```python
from build123d import *

# Parameters (mm, degrees)
SKETCH1_W           = 42.1
SKETCH1_H           = 42.1
BOSS_EXTRUDE1_DEPTH = 32.4
SKETCH2_W           = 17
SKETCH2_H           = 8.5
BOSS_EXTRUDE2_DEPTH = 7.9
BOSS_EXTRUDE3_DEPTH = 7.15
BOSS_EXTRUDE4_DEPTH = 7.2
SKETCH6_R           = 1.5
CUT_EXTRUDE1_DEPTH  = 7.2
CUT_EXTRUDE2_DEPTH  = 7.2
SKETCH9_R           = 6.55
BOSS_EXTRUDE5_DEPTH = 14.6
SKETCH11_R          = 9
BOSS_EXTRUDE6_DEPTH = 6.1
SKETCH12_W          = 17
SKETCH12_H          = 2.5
CUT_EXTRUDE3_DEPTH  = 6
CUT_EXTRUDE4_DEPTH  = 40


with BuildPart() as part:
    # Sketch1 → Boss-Extrude1 (new body)
    with BuildSketch(Plane.XY):
        with Locations((-21.05, 21.05)):
            Rectangle(SKETCH1_W, SKETCH1_H)
    extrude(amount=BOSS_EXTRUDE1_DEPTH)

    # Sketch2 → Boss-Extrude2 (add)
    with BuildSketch(Plane(origin=(0, 42.1, 0), x_dir=(1, 0, 0), z_dir=(0, 1, 0))):
        with Locations((-21.05, -4.25)):
            Rectangle(SKETCH2_W, SKETCH2_H)
    extrude(amount=BOSS_EXTRUDE2_DEPTH)

    # Sketch3 → Boss-Extrude3 (add)
    with BuildSketch(Plane(origin=(0, 0, 0), x_dir=(0, 0, -1), z_dir=(1, 0, 0))):
        Polygon((-32.4, 21.05), (-32.4, 29.05), (-30.8, 29.05), (-30.8, 21.05), (-30.8, 13.05), (-32.4, 13.05), align=None)
    extrude(amount=BOSS_EXTRUDE3_DEPTH)

    # Sketch4 → Boss-Extrude4 (add)
    with BuildSketch(Plane.ZY.offset(42.1)):
        Polygon((32.4, 21.05), (32.4, 29.05), (30.8, 29.05), (30.8, 21.05), (30.8, 13.05), (32.4, 13.05), align=None)
    extrude(amount=BOSS_EXTRUDE4_DEPTH)

    # Sketch6 → Cut-Extrude1 (cut)
    with BuildSketch(Plane.XY.offset(32.4)):
        with Locations((-46.3, 21.060702299)):
            Circle(SKETCH6_R)
        with Locations((4.15, 21.060702299)):
            Circle(SKETCH6_R)
    extrude(amount=-CUT_EXTRUDE1_DEPTH, mode=Mode.SUBTRACT)

    # Sketch7 → Cut-Extrude2 (cut)
    with BuildSketch(Plane.XY.offset(32.4)):
        with BuildLine():
            Line((-42.1, 29.05), (-48.297247635, 23.163320163))
            ThreePointArc((-48.297247635, 23.163320163), (-49.19999881, 21.063329654), (-48.301054234, 18.961706835))
            Line((-48.301054234, 18.961706835), (-42.1, 13.05))
            Line((-42.1, 13.05), (-49.3, 13.05))
            Line((-49.3, 13.05), (-49.3, 29.05))
            Line((-49.3, 29.05), (-42.1, 29.05))
        make_face()
        with BuildLine():
            Line((0, 29.05), (6.155732332, 23.155227976))
            ThreePointArc((6.155732332, 23.155227976), (7.049998812, 21.063327019), (6.159520454, 18.969810731))
            Line((6.159520454, 18.969810731), (0, 13.05))
            Line((0, 13.05), (7.15, 13.05))
            Line((7.15, 13.05), (7.15, 29.05))
            Line((7.15, 29.05), (0, 29.05))
        make_face()
    extrude(amount=-CUT_EXTRUDE2_DEPTH, mode=Mode.SUBTRACT)

    # Sketch9 → Boss-Extrude5 (add)
    with BuildSketch(Plane.XY.offset(32.4)):
        with Locations(Location((-21, 21.05, 0), (0, 0, 180))):
            Circle(SKETCH9_R)
    extrude(amount=BOSS_EXTRUDE5_DEPTH)

    # Sketch11 → Boss-Extrude6 (add)
    with BuildSketch(Plane.XY.offset(32.4)):
        with Locations((-21, 21.05)):
            Circle(SKETCH11_R)
    extrude(amount=BOSS_EXTRUDE6_DEPTH)

    # Sketch12 → Cut-Extrude3 (cut)
    with BuildSketch(Plane(origin=(0, 50, 0), x_dir=(1, 0, 0), z_dir=(0, 1, 0))):
        with Locations((-21.05, -1.25)):
            Rectangle(SKETCH12_W, SKETCH12_H)
    extrude(amount=-CUT_EXTRUDE3_DEPTH, mode=Mode.SUBTRACT)

    # Sketch13 → Cut-Extrude4 (cut)
    with BuildSketch(Plane(origin=(0, 0, 0), x_dir=(-1, 0, 0), z_dir=(0, 0, -1))):
        with BuildLine():
            Line((0, 0), (0, 4))
            ThreePointArc((0, 4), (1.171572875, 1.171572875), (4, 0))
            Line((4, 0), (0, 0))
        make_face()
        with BuildLine():
            Line((38.1, 0), (42.1, 0))
            Line((42.1, 0), (42.1, 4))
            ThreePointArc((42.1, 4), (40.928427125, 1.171572875), (38.1, 0))
        make_face()
        with BuildLine():
            Line((38.1, 42.1), (42.1, 42.1))
            Line((42.1, 42.1), (42.1, 38.1))
            ThreePointArc((42.1, 38.1), (40.928427125, 40.928427125), (38.1, 42.1))
        make_face()
        with BuildLine():
            Line((4, 42.1), (0, 42.1))
            Line((0, 42.1), (0, 38.1))
            ThreePointArc((0, 38.1), (1.171572875, 40.928427125), (4, 42.1))
        make_face()
    extrude(amount=-CUT_EXTRUDE4_DEPTH, mode=Mode.SUBTRACT)


solid = part.part
```
Verification items for the finished model (mm, model axes). A direction names the side the tool comes from. Give positions to 0.01 mm unless a question says otherwise; leave off trailing zeros. Order: outer loops, then holes, each group sorted by start corner. A loop starts at its lowest first (then second) coordinate and runs counter-clockwise, first axis right, second up. Notation, with made-up numbers: (64.25, -26) - (78.25, -26) arc R31 cw to (78.25, 10) - close; hole circle Ø1 at (-4.75, -27.5). An arc over 180 degrees is marked (long way). Answer as CSV lines item,"result". Start each with the question number.
Item 1: Section check C-C, the plane x = -21. Record the boundary of the cut face in (y, z).
Item 2: Material ranges on L1, parallel to Z at x = -5, y = 36.5; L2, parallel to Y at x = -46, z = 31; L3, parallel to Y at x = 4.15, z = 31.9, recorded low to high.
Item 3: Section check D-D, the plane y = 24. Record the boundary of the cut face in (x, z), plus the area to 3 significant figures.
Item 4: Mould release check, pull along X, two halves, no side actions. Record for faces 4 (the face through (-40.959, 40.897, 15.973)), 5 (the face through (3.035, 26.144, 31.611)), 6 (the face through (-47.49, 20.15, 31.61)), 7 (the face through (-21, 21, 47)): released by +X, released by -X, zero draft, split by the parting line, or undercut.
Item 5: Section check B-B, the plane z = 28.5. Record the boundary of the cut face in (x, y), plus the area to 3 significant figures.
Item 6: Section check A-A, the plane x = 4.15. Record the boundary of the cut face in (y, z), plus the area to 3 significant figures.
Item 7: Access from +Z, -Z, +X, -X, +Y, -Y to the whole of each face (thin tool, end or side, straight path). Record for faces 1 (the face through (-21, 47, 2.5)), 2 (the face through (-21, 46, 8.5)), 3 (the face through (-16.847, 13.065, 35.407)).
Item 8: Gauge pin test, flat ends, axial feed: pin 1 (9.5 mm diameter, centred on y = 19.5, z = 19, fed in from +X); pin 2 (2.5 mm diameter, centred on y = 44.5, z = 4.5, fed in from +X); pin 3 (0.8 mm diameter, centred on x = -20, z = 1, fed in from +Y); pin 4 (2.5 mm diameter, centred on x = -46.3, y = 21.06, fed in from -Z). Record the tip position at first contact, or that the pin passes through.
Filled in:
1,outline,"(0, 0) - (44, 0) - (44, 2.5) - (50, 2.5) - (50, 8.5) - (42.1, 8.5) - (42.1, 32.4) - (30.05, 32.4) - (30.05, 38.5) - (27.6, 38.5) - (27.6, 47) - (14.5, 47) - (14.5, 38.5) - (12.05, 38.5) - (12.05, 32.4) - (0, 32.4) - close"
2,L1,"0 to 32.4"
2,L2,"16.77 to 19.59, 22.53 to 25.35"
2,L3,"17.04 to 19.56, 22.56 to 25.08"
3,outline,"(-47.42, 30.8) - (-42.1, 30.8) - (-42.1, 0) - (0, 0) - (0, 30.8) - (5.27, 30.8) - (5.27, 32.4) - (-12.5, 32.4) - (-12.5, 38.5) - (-15.15, 38.5) - (-15.15, 47) - (-26.85, 47) - (-26.85, 38.5) - (-29.5, 38.5) - (-29.5, 32.4) - (-47.42, 32.4) - close"
3,area,"1,580 mm^2"
4,face 4,"released by -X"
4,face 5,"released by +X"
4,face 6,"undercut"
4,face 7,"zero draft"
5,outline,"(-42.1, 4) arc R4 ccw to (-38.1, 0) - (-4, 0) arc R4 ccw to (0, 4) - (0, 38.1) arc R4 ccw to (-4, 42.1) - (-38.1, 42.1) arc R4 ccw to (-42.1, 38.1) - close"
5,area,"1,760 mm^2"
6,outline,"(17.04, 30.8) - (19.56, 30.8) - (19.56, 32.4) - (17.04, 32.4) - close; (22.56, 30.8) - (25.08, 30.8) - (25.08, 32.4) - (22.56, 32.4) - close"
6,area,"8.06 mm^2"
7,face 1,"-Z, +X, -X, +Y"
7,face 2,"+Z, +X, -X, +Y"
7,face 3,"+Z"
8,pin 1,"x = 0"
8,pin 2,"x = -12.55"
8,pin 3,"y = 44"
8,pin 4,"through"
